```python
from build123d import *

# Parameters (mm, degrees)
F0_W      = 158
F0_H      = 115
F1_DEPTH  = 2
F2_W      = 9
F2_H      = 2
F3_DEPTH  = 2
F4_R      = 1
F17_W     = 1.5
F17_H     = 2.5
F18_DEPTH = 2
F19_W     = 20
F19_H     = 14
F20_DEPTH = 2
F22_DEPTH = 25


with BuildPart() as f1:
    # F0 (on Top) → F1 (new body)
    with BuildSketch(Plane.XY):
        with Locations((-98.6276573709, -38.6981162429)):
            Rectangle(F0_W, F0_H)
    extrude(amount=F1_DEPTH)

    # F2 (on face) → F3 (join)
    with BuildSketch(Plane.XY.offset(2)):
        Polygon((-155.1276573709, 16.8018837571), (-175.6276573709, 16.8018837571), (-175.6276573709, -94.1981162429), (-125.6276573709, -94.1981162429), (-125.6276573709, 16.8018837571), (-146.1276573709, 16.8018837571), align=None)
        with Locations((-150.6276573709, 17.8018837571)):
            Rectangle(F2_W, F2_H)
        Polygon((-103.1276573709, 16.8018837571), (-123.6276573709, 16.8018837571), (-123.6276573709, -94.1981162429), (-73.6276573709, -94.1981162429), (-73.6276573709, 16.8018837571), (-94.1276573709, 16.8018837571), align=None)
        with Locations((-98.6276573709, 17.8018837571)):
            Rectangle(F2_W, F2_H)
        Polygon((-51.1276573709, 16.8018837571), (-71.6276573709, 16.8018837571), (-71.6276573709, -94.1981162429), (-21.6276573709, -94.1981162429), (-21.6276573709, 16.8018837571), (-42.1276573709, 16.8018837571), align=None)
        with Locations((-46.6276573709, 17.8018837571)):
            Rectangle(F2_W, F2_H)
    extrude(amount=F3_DEPTH)

    # F4
    f4_edges = [f1.edges().sort_by_distance(p)[0] for p in [
        (-150.627657, 18.801884, 4),
        (-98.627657, 18.801884, 4),
        (-46.627657, 18.801884, 4),
    ]]
    fillet(f4_edges, radius=F4_R)

    # F5 (on face) → F6 (revolve, cut)
    with BuildSketch(Plane(origin=(-155.1276573709, 0, 0), x_dir=(0, -1, 0), z_dir=(-1, 0, 0))):
        with BuildLine():
            Line((-18.2392987821, 2.3907643347), (-17.368703077, 3.6122536226))
            ThreePointArc((-17.368703077, 3.6122536226), (-18.4126320707, 3.435300468), (-18.2392987821, 2.3907643347))
        make_face()
    revolve(axis=Axis((-155.1276573709, 17.8040009295, 3.0015089786), (0, -0.580400624, 0.8143310848)), mode=Mode.SUBTRACT)

    # F7 (on face) → F8 (revolve, cut)
    with BuildSketch(Plane.YZ.offset(-146.1276573709)):
        with BuildLine():
            ThreePointArc((18.497534939, 2.719697604), (18.5381711964, 2.8572386368), (18.5518837571, 3))
            ThreePointArc((18.5518837571, 3), (17.9358816289, 3.7379326327), (17.0997649028, 3.2636837395))
            Line((17.0997649028, 3.2636837395), (18.497534939, 2.719697604))
        make_face()
    revolve(axis=Axis((-146.1276573709, 17.7986499209, 2.9916906717), (0, -0.9319125504, 0.362683055)), mode=Mode.SUBTRACT)

    # F9 (on face) → F10 (revolve, cut)
    with BuildSketch(Plane(origin=(-103.1276573709, 0, 0), x_dir=(0, -1, 0), z_dir=(-1, 0, 0))):
        with BuildLine():
            Line((-18.2199622799, 2.3773360868), (-17.3826746537, 3.6219033105))
            ThreePointArc((-17.3826746537, 3.6219033105), (-18.4241676257, 3.4186439858), (-18.2199622799, 2.3773360868))
        make_face()
    revolve(axis=Axis((-103.1276573709, 17.8013184668, 2.9996196986), (0, -0.5581919811, 0.8297118248)), mode=Mode.SUBTRACT)

    # F11 (on face) → F12 (revolve, cut)
    with BuildSketch(Plane.YZ.offset(-94.1276573709)):
        with BuildLine():
            ThreePointArc((18.1709835579, 2.3471100115), (18.4496973301, 2.6220614141), (18.5518837571, 3))
            ThreePointArc((18.5518837571, 3), (18.1802362306, 3.647571931), (17.4336186749, 3.6533611782))
            Line((17.4336186749, 3.6533611782), (18.1709835579, 2.3471100115))
        make_face()
    revolve(axis=Axis((-94.1276573709, 17.8023011164, 3.0002355949), (0, -0.4915766891, 0.8708342889)), mode=Mode.SUBTRACT)

    # F13 (on face) → F14 (revolve, cut)
    with BuildSketch(Plane(origin=(-51.1276573709, 0, 0), x_dir=(0, -1, 0), z_dir=(-1, 0, 0))):
        with BuildLine():
            Line((-18.4692159742, 2.6577023049), (-17.133300999, 3.3398486363))
            ThreePointArc((-17.133300999, 3.3398486363), (-18.1429574959, 3.66795861), (-18.4692159742, 2.6577023049))
        make_face()
    revolve(axis=Axis((-51.1276573709, 17.8012584866, 2.9987754706), (0, -0.89061148, 0.4547649851)), mode=Mode.SUBTRACT)

    # F15 (on face) → F16 (revolve, cut)
    with BuildSketch(Plane.YZ.offset(-42.1276573709)):
        with BuildLine():
            Line((18.5518387793, 2.9917863059), (17.051928735, 2.9917863059))
            ThreePointArc((17.051928735, 2.9917863059), (17.8018837571, 2.25), (18.5518387793, 2.9917863059))
        make_face()
    revolve(axis=Axis((-42.1276573709, 17.8018837571, 2.9917863059), (0, -1, 0)), mode=Mode.SUBTRACT)

    # F17 (on face) → F18 (cut)
    with BuildSketch(Plane.XY.offset(4)):
        with Locations((-174.8776573709, 15.5518837571)):
            Rectangle(F17_W, F17_H)
        with Locations((-174.8776573709, -92.9481162429)):
            Rectangle(F17_W, F17_H)
    extrude(amount=-F18_DEPTH, mode=Mode.SUBTRACT)

    # F19 (on face) → F20 (join, symmetric)
    with BuildSketch(Plane.XZ.offset(96.1981162429)):
        with Locations((-98.6276573709, 7)):
            Rectangle(F19_W, F19_H)
    extrude(amount=F20_DEPTH, both=True)

    # F21 (on face) → F22 (cut)
    with BuildSketch(Plane(origin=(-108.6276573709, 0, 0), x_dir=(0, -1, 0), z_dir=(-1, 0, 0))):
        Polygon((94.1981162429, 12), (94.1981162429, 2), (96.1981162429, 2), (96.1981162429, 12), (95.1981162429, 12), align=None)
        Polygon((94.1981162429, 14), (94.1981162429, 12), (95.1981162429, 12), (98.1981162429, 14), align=None)
    extrude(amount=-F22_DEPTH, mode=Mode.SUBTRACT)


solid = f1.part
```
Can you work these out from the model? Positions are in its coordinate system, mm. A direction names the side the tool comes from. Coordinates: 2 decimals unless noted, no trailing zeros. Write each loop counter-clockwise with the first axis right and the second up, starting at its lowest first coordinate (ties: lowest second). Pieces come first, ordered by that corner, then holes. Notation, with made-up numbers: M 63.5,73 L 96.5,73 A18 cw 96.5,77 Z; hole C 49.25,69.5 d8. An arc over 180 degrees is marked long. Answer as CSV lines item,"result".
Item 1: We'd pull the mould along Z, two halves only. Please class faces 3 (the flat face through (-100, -39, 0)), 4 (the flat face through (-99, -96.198, 7)), 5 (the flat face through (-47, -37, 4)), 6 (the flat face through (-99, -98.198, 7)): +Z half, -Z half, draft (parallel to the pull), parting line (faces both ways), or undercut.
Geometry results:
face 3,"-Z half"
face 4,"undercut"
face 5,"+Z half"
face 6,"draft"
Item 2: On a 3-axis mill with a long thin cutter (end or side, diameter ignored), from which of +Z, -Z, +X, -X, +Y, -Y can I reach the whole of each face in a straight line? I mean faces 1 (the flat face through (-99, -37, 4)), 2 (the flat face through (-100, 18.802, 1)). Say none if no direction works.
Geometry results:
face 1,"+Z, +X, -X, +Y"
face 2,"+Z, -Z, +X, -X, +Y"
Item 3: Please list where these lines run through material, in increasing order: line 1 along X through (y, z) = (-68, 3.75); line 2 along Z through (x, y) = (-45, -48); line 3 along Y through (x, z) = (-155, 0.75).
Geometry results:
line 1,"x = -175.63 to -125.63, -123.63 to -73.63, -71.63 to -21.63"
line 2,"z = 0 to 4"
line 3,"y = -96.2 to 18.8"
Item 4: Imagine slicing it at B-B on x = -136.5. List the corners of the cut face in (y, z) for me, plus the area to 3 significant figures.
Geometry results:
outline,"M -96.2,0 L 18.8,0 L 18.8,2 L 16.8,2 L 16.8,4 L -94.2,4 L -94.2,2 L -96.2,2 Z"
area,"452 mm2"
Item 5: I'm going to push flat-ended pins straight in: P1, Ø2, axis at x = -62, z = 3.5, coming from the +Y side; P2, Ø6, axis at y = -74.5, z = 6, coming from the -X side; P3, Ø1.6, axis at x = -175, z = 3, coming from the -Y side; P4, Ø4, axis at y = -61.5, z = 7, coming from the -X side. Where does each tip first touch, or does it pass through?
Geometry results:
P1,"stops at y = 16.8"
P2,"stops at x = -175.63"
P3,"stops at y = -91.7"
P4,"passes through"
Item 6: Imagine slicing it at C-C on z = 8. List the corners of the cut face in (x, y) for me.
Geometry results:
outline,"M -108.63,-98.2 L -88.63,-98.2 L -88.63,-96.2 L -108.63,-96.2 Z"
Item 7: Imagine slicing it at A-A on y = 10. List the corners of the cut face in (x, z) for me, plus the area to 3 significant figures.
Geometry results:
outline,"M -177.63,0 L -19.63,0 L -19.63,2 L -21.63,2 L -21.63,4 L -71.63,4 L -71.63,2 L -73.63,2 L -73.63,4 L -123.63,4 L -123.63,2 L -125.63,2 L -125.63,4 L -175.63,4 L -175.63,2 L -177.63,2 Z"
area,"616 mm2"
